Design review of the part built by this model. Coordinates are the model's own, in mm. Round coordinates to 2 decimals unless told otherwise and drop trailing zeros. Order: outer loops, then holes, each group sorted by start corner. A loop starts at its lowest first (then second) coordinate and runs counter-clockwise, first axis right, second up. Notation, with made-up numbers: M 28.25,19.5 L 83.25,19.5 A36 ccw 83.25,58.5 Z; hole C 18,46.25 d1. An arc over 180 degrees is marked long. Write item = value, one per line. Start each with the question number.
```python
from build123d import *

# Parameters (mm, degrees)
F1_DEPTH = 2
F3_D     = 2.4
F4_R     = 3


with BuildPart() as f1:
    # F0 (on Top) → F1 (new body)
    with BuildSketch(Plane.XY):
        Polygon((25, 43.3012701892), (-25, 43.3012701892), (-50, 0), (-25, -43.3012701892), (25, -43.3012701892), (50, 0), align=None)
    extrude(amount=F1_DEPTH)

    # F3 (through all)
    with Locations(Plane.XY.offset(2)):
        with Locations((-18, 31.1769145362), (18, 31.1769145362), (36, 0), (18, -31.1769145362), (-18, -31.1769145362), (-36, 0)):
            Hole(F3_D / 2)

    # F4
    f4_edges = [f1.edges().sort_by_distance(p)[0] for p in [
        (-25, -43.30127, 1),
        (25, -43.30127, 1),
        (50, 0, 1),
        (25, 43.30127, 1),
        (-25, 43.30127, 1),
        (-50, 0, 1),
    ]]
    fillet(f4_edges, radius=F4_R)


solid = f1.part
```
(1) For line 1 along Y through (x, z) = (-18, 1.25); line 2 along X through (y, z) = (31.5, 0.9); line 3 along Y through (x, z) = (36, 0.85), list the stretches that pass through material, from the lowest coordinate up. Write a range as [from, to].
(2) Insertion check: pin 1 (1.4 mm diameter, centred on x = -18, y = -31.18, fed in from -Z); pin 2 (1 mm diameter, centred on y = -11, z = 1.5, fed in from +X). Each pin has a flat end and moves straight along its axis. Give the tip position at first contact, or say it passes through.
(3) Draft analysis for pull direction Y (two halves, no side actions). For faces 1 (the face through (18.156, -29.987, 0.986)), 2 (the face through (-24.787, -42.888, 1.014)), 3 (the face through (-1, 1, 2)), state which applies: pulls with the +Y half, pulls with the -Y half, needs draft (parallel to the pull), parting line crosses it, or undercut.
(4) Consider section D-D, the plane x = 36. Write out the cut boundary in (y, z).
(5) Consider section C-C, the plane z = 0.95. Write out the cut boundary in (x, y), then the cut area to 3 significant figures.
(6) Consider section A-A, the plane y = 0. Write out the cut boundary in (x, z), then the cut area to 3 significant figures.
(7) Consider section B-B, the plane x = -18. Write out the cut boundary in (y, z).
Completed:
q1.line_1 = [-43.3, -32.38], [-29.98, 29.98], [32.38, 43.3]
q1.line_2 = [-31.81, -19.16], [-16.84, 16.84], [19.16, 31.81]
q1.line_3 = [-24.25, -1.2], [1.2, 24.25]
q2.pin_1 = through
q2.pin_2 = 43.94
q3.face_1 = undercut
q3.face_2 = pulls with the -Y half
q3.face_3 = needs draft
q4.outline = M -24.25,0 L -1.2,0 L -1.2,2 L -24.25,2 Z; M 1.2,0 L 24.25,0 L 24.25,2 L 1.2,2 Z
q5.outline = M -49.13,-1.5 L -25.87,-41.8 A3 ccw -23.27,-43.3 L 23.27,-43.3 A3 ccw 25.87,-41.8 L 49.13,-1.5 A3 ccw 49.13,1.5 L 25.87,41.8 A3 ccw 23.27,43.3 L -23.27,43.3 A3 ccw -25.87,41.8 L -49.13,1.5 A3 ccw Z; hole C -36,0 d2.4; hole C -18,-31.18 d2.4; hole C -18,31.18 d2.4; hole C 18,-31.18 d2.4; hole C 18,31.18 d2.4; hole C 36,0 d2.4
q5.area = 6,470 mm2
q6.outline = M -49.54,0 L -37.2,0 L -37.2,2 L -49.54,2 Z; M -34.8,0 L 34.8,0 L 34.8,2 L -34.8,2 Z; M 37.2,0 L 49.54,0 L 49.54,2 L 37.2,2 Z
q6.area = 189 mm2
q7.outline = M -43.3,0 L -32.38,0 L -32.38,2 L -43.3,2 Z; M -29.98,0 L 29.98,0 L 29.98,2 L -29.98,2 Z; M 32.38,0 L 43.3,0 L 43.3,2 L 32.38,2 Z
